Part model, mm, in its own coordinate system. Coordinates: 2 decimals unless noted, no trailing zeros. Order: outer loops, then holes, each group sorted by start corner. A loop starts at its lowest first (then second) coordinate and runs counter-clockwise, first axis right, second up. Notation, with made-up numbers: (51, 10.5) - (60, 10.5) arc R20 ccw to (60, 31.5) - close; hole circle Ø2 at (-39.5, -24). An arc over 180 degrees is marked (long way). Use a Markdown table: item, result. Add a question column.
1) Drop flat-ended pins along their axis: P1, Ø15, axis at x = 37, z = -39.5, coming from the -Y side; P2, Ø2, axis at x = 18, y = 50.5, coming from the +Z side; P3, Ø4, axis at x = 24.5, y = 48.5, coming from the +Z side. Give the stop position or say it passes through.
2) Saw through at A-A on y = 7.5. List the corners of the cut face in (x, z).
3) Saw through at C-C on z = -33. List the corners of the cut face in (x, y).
4) Saw through at D-D on y = 25.5. List the corners of the cut face in (x, z).
5) Saw through at B-B on x = 65.5. List the corners of the cut face in (y, z), then the cut area to 3 significant figures.
6) Wall check: L1, parallel to Y at x = 28, z = -41; L2, parallel to X at y = 31.5, z = -31.5; L3, parallel to X at y = 48, z = -11. Give the ranges that are in metal, low to high. Write a range as [from, to].
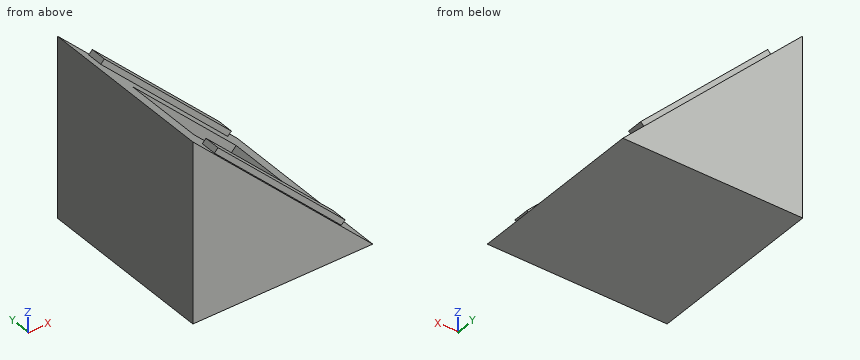
```python
from build123d import *

# Parameters (mm, degrees)
SKETCH1_W           = 69.85
SKETCH1_H           = 69.85
BOSS_EXTRUDE1_DEPTH = 69.85
CUT_EXTRUDE2_DEPTH  = 100
SKETCH3_W           = 69.723
SKETCH3_H           = 6.223
BOSS_EXTRUDE2_DEPTH = 2.032
SKETCH4_W           = 57.15
SKETCH4_H           = 31.75
CUT_EXTRUDE3_DEPTH  = 12.7


with BuildPart() as part:
    # Sketch1 → Boss-Extrude1 (new body)
    with BuildSketch(Plane(origin=(0, 0, 0), x_dir=(1, 0, 0), z_dir=(0, 1, 0))):
        with Locations((34.925, 34.925)):
            Rectangle(SKETCH1_W, SKETCH1_H)
    extrude(amount=BOSS_EXTRUDE1_DEPTH)

    # Sketch2 → Cut-Extrude2 (cut)
    with BuildSketch(Plane(origin=(0, 0, 0), x_dir=(0.707106781, 0, -0.707106781), z_dir=(0.707106781, 0, 0.707106781))):
        Polygon((98.782817332, 69.85), (98.782817332, 0), (49.391408666, 0), (0, 0), (0, 69.85), (49.391408666, 69.85), align=None)
    extrude(amount=CUT_EXTRUDE2_DEPTH, mode=Mode.SUBTRACT)

    # Sketch3 → Boss-Extrude2 (add)
    with BuildSketch(Plane(origin=(0, 0, 0), x_dir=(0.707106781, 0, -0.707106781), z_dir=(0.707106781, 0, 0.707106781))):
        with Locations((49.391408666, 5.6515)):
            Rectangle(SKETCH3_W, SKETCH3_H)
        with Locations((49.391408666, 64.1985)):
            Rectangle(SKETCH3_W, SKETCH3_H)
    extrude(amount=BOSS_EXTRUDE2_DEPTH)

    # Sketch4 → Cut-Extrude3 (cut)
    with BuildSketch(Plane(origin=(0, 0, 0), x_dir=(0.707106781, 0, -0.707106781), z_dir=(0.707106781, 0, 0.707106781))):
        with Locations((49.391408666, 34.925)):
            Rectangle(SKETCH4_W, SKETCH4_H)
    extrude(amount=-CUT_EXTRUDE3_DEPTH, mode=Mode.SUBTRACT)


solid = part.part
```
Results are:
| question | item | result |
|---|---|---|
| 1 | P1 | y = 0 |
| 1 | P2 | z = -17.05 |
| 1 | P3 | z = -40.46 |
| 2 | outline | (0, -69.85) - (69.85, -69.85) - (59.58, -59.58) - (61.01, -58.14) - (11.71, -8.84) - (10.27, -10.27) - (0, 0) - close |
| 3 | outline | (0, 0) - (33, 0) - (33, 2.54) - (35.87, 2.54) - (35.87, 8.76) - (33, 8.76) - (33, 19.05) - (15.04, 19.05) - (15.04, 50.8) - (33, 50.8) - (33, 61.09) - (35.87, 61.09) - (35.87, 67.31) - (33, 67.31) - (33, 69.85) - (0, 69.85) - close |
| 4 | outline | (0, -69.85) - (69.85, -69.85) - (55.13, -55.13) - (46.15, -64.11) - (5.74, -23.7) - (14.72, -14.72) - (0, 0) - close |
| 5 | outline | (0, -69.85) - (69.85, -69.85) - (69.85, -65.5) - (0, -65.5) - close |
| 5 | area | 304 mm2 |
| 6 | L1 | [0, 19.05], [50.8, 69.85] |
| 6 | L2 | [0, 13.54] |
| 6 | L3 | [0, 11] |
